Part print with two shaded views. Sizes in mm from the minimum x, y, z corner. Coordinates: 2 decimals unless noted, no trailing zeros. Write each loop counter-clockwise with the first axis right and the second up, starting at its lowest first coordinate (ties: lowest second). Pieces come first, ordered by that corner, then holes.
Q1. Band-saw the part on A-A, the plane x = 173. Write the cut outline in (y, z).
Q2. Band-saw the part on C-C, the plane z = 0.75. Write the cut outline in (x, y), plus the area to 3 significant figures.
Q3. Drill centre lines: probe 1 along X at (y, z) = (140, 3.15); probe 2 along Y at (x, z) = (137, 3.3); probe 3 along X at (y, z) = (132, 0.45) (1 decimal). Where is each one in solid material? Low to high.
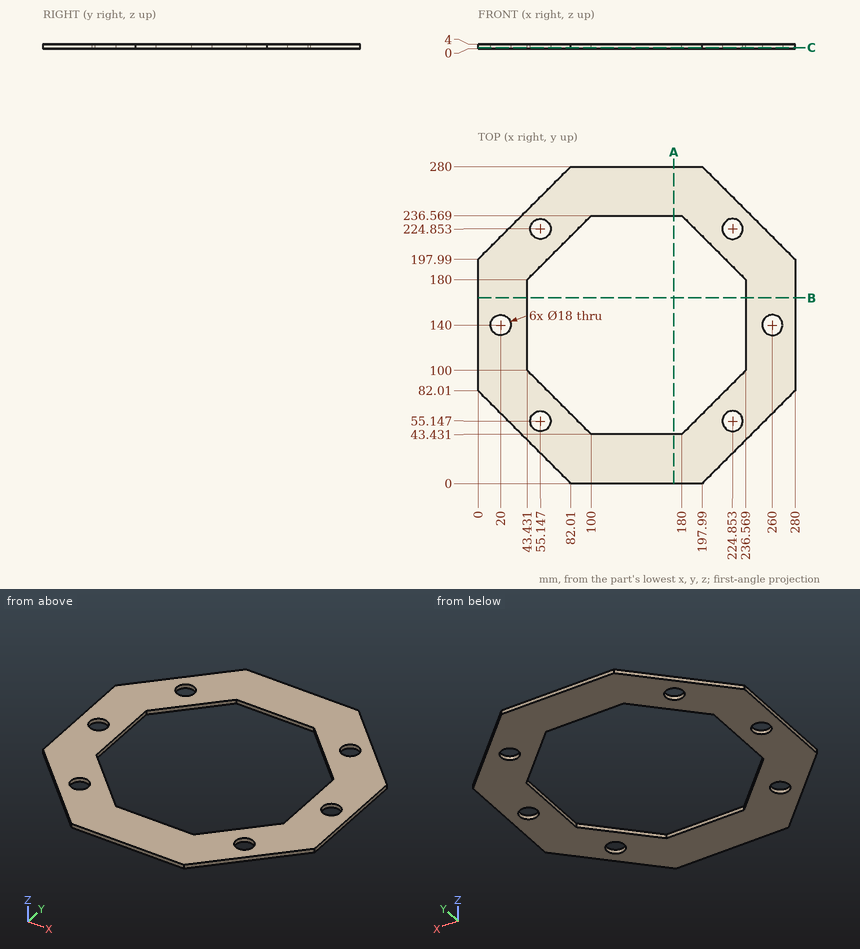
Answer sheet:
1. outline: (0, 0) - (43.43, 0) - (43.43, 4) - (0, 4) - close; (236.57, 0) - (280, 0) - (280, 4) - (236.57, 4) - close
2. outline: (0, 82.01) - (82.01, 0) - (197.99, 0) - (280, 82.01) - (280, 197.99) - (197.99, 280) - (82.01, 280) - (0, 197.99) - close; hole circle Ø18 at (20, 140); hole (43.43, 100) - (100, 43.43) - (180, 43.43) - (236.57, 100) - (236.57, 180) - (180, 236.57) - (100, 236.57) - (43.43, 180) - close; hole circle Ø18 at (55.15, 55.15); hole circle Ø18 at (55.15, 224.85); hole circle Ø18 at (224.85, 55.15); hole circle Ø18 at (224.85, 224.85); hole circle Ø18 at (260, 140)
2. area: 32,500 mm2
3. probe 1: x = 0 to 11, 29 to 43.43, 236.57 to 251, 269 to 280
3. probe 2: y = 0 to 43.43, 236.57 to 280
3. probe 3: x = 0 to 15.9, 24.1 to 43.4, 236.6 to 255.9, 264.1 to 280
